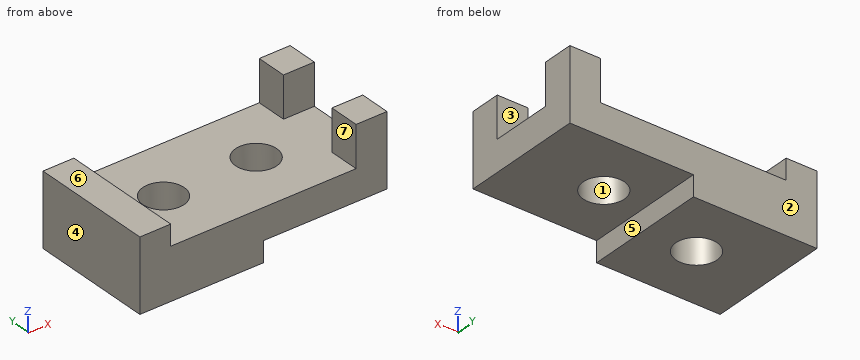
```python
from build123d import *

# Parameters (mm, degrees)
SKETCH_W        = 120
SKETCH_H        = 60
PAD_DEPTH       = 35
SKETCH001_W     = 122.740021
SKETCH001_H     = 89.853363
POCKET_DEPTH    = 10
SKETCH002_W     = 72.220016
SKETCH002_H     = 101.200035
POCKET001_DEPTH = 10
SKETCH003_W     = 15
SKETCH003_H     = 15
PAD001_DEPTH    = 20
SKETCH004_R     = 10
POCKET002_DEPTH = 25.001


with BuildPart() as part:
    # Sketch → Pad (new body)
    with BuildSketch(Plane.XY):
        Rectangle(SKETCH_W, SKETCH_H)
    extrude(amount=PAD_DEPTH)

    # Sketch001 → Pocket (cut)
    with BuildSketch(Plane.XY.offset(35)):
        with Locations((16.37001, -4.44667)):
            Rectangle(SKETCH001_W, SKETCH001_H)
    extrude(amount=-POCKET_DEPTH, mode=Mode.SUBTRACT)

    # Sketch002 → Pocket001 (cut)
    with BuildSketch(Plane(origin=(0, 0, 0), x_dir=(1, 0, 0), z_dir=(0, 0, -1))):
        with Locations((36.110008, 2.760006)):
            Rectangle(SKETCH002_W, SKETCH002_H)
    extrude(amount=-POCKET001_DEPTH, mode=Mode.SUBTRACT)

    # Sketch003 → Pad001 (new body)
    with BuildSketch(Plane.XY.offset(25)):
        with Locations((52.5, 22.5)):
            Rectangle(SKETCH003_W, SKETCH003_H)
        with Locations((52.5, -22.5)):
            Rectangle(SKETCH003_W, SKETCH003_H)
    extrude(amount=PAD001_DEPTH)

    # Sketch004 → Pocket002 (cut, through all)
    with BuildSketch(Plane.XY.offset(25)):
        with Locations((-25, 0)):
            Circle(SKETCH004_R)
        with Locations((20, 0)):
            Circle(SKETCH004_R)
    extrude(amount=-POCKET002_DEPTH, mode=Mode.SUBTRACT)


solid = part.part
```
Here's how the part is built. I have some questions about the finished solid (model axes, mm). Face numbers are marked on the shaded views. A direction names the side the tool comes from. Coordinates: 2 decimals unless noted, no trailing zeros. Order: outer loops, then holes, each group sorted by start corner. A loop starts at its lowest first (then second) coordinate and runs counter-clockwise, first axis right, second up.
1) Which directions (+Z, -Z, +X, -X, +Y, -Y) give clear straight access to the entire face, cutting with the end or side of a thin tool? Please do the marked faces 5, 6 and 7.
2) I need wall thicknesses on line 1 (Y direction, x = -25, z = 6); line 2 (X direction, y = -20, z = 26); line 3 (Z direction, x = 47, y = -19). Which ranges of each line are inside material? Lowest first, please.
3) Imagine slicing it at A-A on y = 0. List the corners of the cut face in (x, z) for me.
4) Imagine slicing it at C-C on z = 38. List the corners of the cut face in (x, y) for me.
5) Will these pins go through, and if not, where does the flat tip stop? pin 1 (5 mm diameter, centred on x = 6.5, z = 28.5, fed in from +Y); pin 2 (10 mm diameter, centred on x = 7.5, y = 20, fed in from -Z); pin 3 (7.5 mm diameter, centred on x = -52, y = 13, fed in from +Z); pin 4 (12 mm diameter, centred on x = -26.5, y = -5, fed in from +Z).
6) Imagine slicing it at B-B on x = 20. List the corners of the cut face in (y, z) for me, and give its area (3 significant figures).
7) Imagine slicing it at D-D on z = 6. List the corners of the cut face in (x, y) for me.
8) We'd pull the mould along Y, two halves only. Please class the marked faces 1, 2, 3 and 4: +Y half, -Y half, draft (parallel to the pull), parting line (faces both ways), or undercut.
Response values:
1. face 5: -Z, +X, +Y, -Y
1. face 6: +Z, -X, +Y, -Y
1. face 7: +Z, +Y, -Y
2. line 1: y = -30 to -10, 10 to 30
2. line 2: x = -60 to -45, 45 to 60
2. line 3: z = 10 to 45
3. outline: (-60, 0) - (-35, 0) - (-35, 25) - (-45, 25) - (-45, 35) - (-60, 35) - close; (-15, 0) - (0, 0) - (0, 10) - (10, 10) - (10, 25) - (-15, 25) - close; (30, 10) - (60, 10) - (60, 25) - (30, 25) - close
4. outline: (45, -30) - (60, -30) - (60, -15) - (45, -15) - close; (45, 15) - (60, 15) - (60, 30) - (45, 30) - close
5. pin 1: passes through
5. pin 2: stops at z = 10
5. pin 3: stops at z = 35
5. pin 4: stops at z = 25
6. outline: (-30, 10) - (-10, 10) - (-10, 25) - (-30, 25) - close; (10, 10) - (30, 10) - (30, 25) - (10, 25) - close
6. area: 600 mm2
7. outline: (-60, -30) - (0, -30) - (0, 30) - (-60, 30) - close; hole circle Ø20 at (-25, 0)
8. face 1: undercut
8. face 2: +Y half
8. face 3: undercut
8. face 4: draft
